```python
from build123d import *

# Parameters (mm, degrees)
F0_R     = 5.5
F1_DEPTH = 2


with BuildPart() as f1:
    # F0 (on Top) → F1 (new body)
    with BuildSketch(Plane.XY):
        with BuildLine():
            Line((15, 23), (-15, 23))
            Line((-15, 23), (-18, 23))
            ThreePointArc((-18, 23), (-20.12132, 22.12132), (-21, 20))
            Line((-21, 20), (-21, -14))
            ThreePointArc((-21, -14), (-20.414214, -15.414214), (-19, -16))
            Line((-19, -16), (-17, -16))
            Line((-17, -16), (-17, -2))
            Line((-17, -2), (-15, -2))
            Line((-15, -2), (-15, -23))
            Line((-15, -23), (15, -23))
            Line((15, -23), (15, -2))
            Line((15, -2), (17, -2))
            Line((17, -2), (17, -16))
            Line((17, -16), (19, -16))
            ThreePointArc((19, -16), (20.414214, -15.414214), (21, -14))
            Line((21, -14), (21, 20))
            ThreePointArc((21, 20), (20.12132, 22.12132), (18, 23))
            Line((18, 23), (15, 23))
        make_face()
        with Locations((-8.5, 10.5)):
            Circle(F0_R, mode=Mode.SUBTRACT)
        with Locations((8.5, 10.5)):
            Circle(F0_R, mode=Mode.SUBTRACT)
    extrude(amount=F1_DEPTH)


solid = f1.part
```
Source: CAD feature listing. Evaluate the final solid. Frame: model axes, mm. A direction names the side the tool comes from. Coordinates: 2 decimals unless noted, no trailing zeros. Write each loop counter-clockwise with the first axis right and the second up, starting at its lowest first coordinate (ties: lowest second). Pieces come first, ordered by that corner, then holes. Notation, with made-up numbers: M 59,-18.75 L 106,-18.75 A20 ccw 106,20.25 Z; hole C 35,33.5 d1. An arc over 180 degrees is marked long. Answer as a JSON object with one key per item and string values.
1. Cut plane C-C on z = 1.5. Output: boundary loops of the cut face in (x, y), plus the area to 3 significant figures.
Evaluation:
{"outline": "M -21,-14 A2 ccw -19,-16 L -17,-16 L -17,-2 L -15,-2 L -15,-23 L 15,-23 L 15,-2 L 17,-2 L 17,-16 L 19,-16 A2 ccw 21,-14 L 21,20 A3 ccw 18,23 L -18,23 A3 ccw -21,20 Z; hole C -8.5,10.5 d11; hole C 8.5,10.5 d11", "area": "1,600 mm^2"}
2. Cut plane B-B on x = -8.5. Output: boundary loops of the cut face in (y, z), plus the area to 3 significant figures.
Evaluation:
{"outline": "M -23,0 L 5,0 L 5,2 L -23,2 Z; M 16,0 L 23,0 L 23,2 L 16,2 Z", "area": "70.0 mm^2"}
3. Cut plane A-A on y = 10.5. Output: boundary loops of the cut face in (x, z), plus the area to 3 significant figures.
Evaluation:
{"outline": "M -21,0 L -14,0 L -14,2 L -21,2 Z; M -3,0 L 3,0 L 3,2 L -3,2 Z; M 14,0 L 21,0 L 21,2 L 14,2 Z", "area": "40.0 mm^2"}
4. Access query for faces 1 (the flat face through (-18, -16, 1)), 2 (the flat face through (17, -9, 1)), 3 (the flat face through (18, -16, 1)). Directions: +Z, -Z, +X, -X, +Y, -Y. A direction counts if a zero-diameter tool reaches every point of the face in a straight line with its end or side. Return the directions, or none.
Evaluation:
{"face 1": "+Z, -Z, -X, -Y", "face 2": "+Z, -Z, -Y", "face 3": "+Z, -Z, +X, -Y"}
5. Ray query, L1, parallel to X at y = -7.5, z = 0.95; L2, parallel to Y at x = -8.5, z = 0.7; L3, parallel to X at y = -17, z = 0.55. Return the intervals inside material, ascending.
Evaluation:
{"L1": "-21 to -17, -15 to 15, 17 to 21", "L2": "-23 to 5, 16 to 23", "L3": "-15 to 15"}
6. Cut plane D-D on x = 6. Output: boundary loops of the cut face in (y, z), plus the area to 3 significant figures.
Evaluation:
{"outline": "M -23,0 L 5.6,0 L 5.6,2 L -23,2 Z; M 15.4,0 L 23,0 L 23,2 L 15.4,2 Z", "area": "72.4 mm^2"}
7. Contact query for flat-ended pins moving along their axis: P1, Ø0.6, axis at x = -16.5, z = 1, coming from the -Y side; P2, Ø0.6, axis at x = -18, z = 1, coming from the -Y side; P3, Ø6.5, axis at x = -8.5, y = 10.5, coming from the +Z side; P4, Ø0.6, axis at y = -16, z = 1, coming from the -X side. Output: stop coordinate, or through.
Evaluation:
{"P1": "y = -2", "P2": "y = -16", "P3": "through", "P4": "x = -20.05"}
8. Draft query along X for faces 4 (the cylindrical face through (20.4, -15.43, 0.99)), 5 (the flat face through (0, -23, 1)), 6 (the cylindrical face through (13.58, 8.39, 0.99)). Return one class per face: released by +X, released by -X, zero draft, split by the parting line, or undercut.
Evaluation:
{"face 4": "released by +X", "face 5": "zero draft", "face 6": "undercut"}
